from build123d import *

# Parameters (mm, degrees)
SKETCH1_W                                         = 6.35
SKETCH1_H                                         = 9.5
BOSS_EXTRUDE1_DEPTH                               = 5.3
SKETCH2_W                                         = 17.283420288
SKETCH2_H                                         = 7.484
BOSS_EXTRUDE2_DEPTH                               = 3.175
SKETCH3_R                                         = 0.954
CUT_EXTRUDE1_DEPTH                                = 16.91379719
SKETCH4_W                                         = 6.35
SKETCH4_H                                         = 1.008
BOSS_EXTRUDE3_DEPTH                               = 3.175
CHAMFER1_SIZE                                     = 3.175
CHAMFER2_SIZE                                     = 1.5875
CHAMFER3_SIZE                                     = 0.762
CSK_FOR_4_FLAT_HEAD_MACHINE_SCREW_100_D           = 3.4544
CSK_FOR_4_FLAT_HEAD_MACHINE_SCREW_100_CSINK_D     = 5.715
CSK_FOR_4_FLAT_HEAD_MACHINE_SCREW_100_CSINK_ANGLE = 100


with BuildPart() as part:
    # Sketch1 → Boss-Extrude1 (new body)
    with BuildSketch(Plane.XY):
        with Locations((9.429, 0)):
            Rectangle(SKETCH1_W, SKETCH1_H)
    extrude(amount=BOSS_EXTRUDE1_DEPTH)

    # Sketch2 → Boss-Extrude2 (add)
    with BuildSketch(Plane.XY.offset(5.3)):
        with Locations((3.962289856, 0)):
            Rectangle(SKETCH2_W, SKETCH2_H)
    extrude(amount=BOSS_EXTRUDE2_DEPTH)

    # Sketch3 → Cut-Extrude1 (cut, through all)
    with BuildSketch(Plane.XY.offset(8.475)):
        with Locations((-4, 0)):
            Circle(SKETCH3_R)
        with Locations((3.5, 0)):
            Circle(SKETCH3_R)
    extrude(amount=-CUT_EXTRUDE1_DEPTH, mode=Mode.SUBTRACT)

    # Sketch4 → Boss-Extrude3 (add)
    with BuildSketch(Plane.XY.offset(5.3)):
        with Locations((9.429, 4.246)):
            Rectangle(SKETCH4_W, SKETCH4_H)
        with Locations((9.429, -4.246)):
            Rectangle(SKETCH4_W, SKETCH4_H)
    extrude(amount=BOSS_EXTRUDE3_DEPTH)

    # Chamfer1
    # the kernel refuses this chamfer: 3.175 mm, written as the material it adds along each edge
    with BuildSketch(Plane(origin=(6.254, 3.742, 5.3), x_dir=(-0.9996219169112968, -0.027495876610586466, 0), z_dir=(0, 0, 1))) as chamfer1_piece_1_section:
        Polygon((CHAMFER1_SIZE * 0.999621916911, -CHAMFER1_SIZE * 0.0274958766106), (-CHAMFER1_SIZE * 0.0274958766106, -CHAMFER1_SIZE * 0.999621916911), (0, 0), align=None)
    chamfer1_piece_1 = extrude(amount=3.175, mode=Mode.PRIVATE)
    chamfer1_piece_1 = split(chamfer1_piece_1, bisect_by=Plane(origin=(4.881200971, 4.75, 6.8875), z_dir=(0, -1, 0)), keep=Keep.TOP, mode=Mode.PRIVATE)
    add(chamfer1_piece_1)
    with BuildSketch(Plane(origin=(6.254, -3.742, 5.3), x_dir=(-0.9996219169112968, 0.027495876610586324, 0), z_dir=(0, 0, 1))) as chamfer1_piece_2_section:
        Polygon((CHAMFER1_SIZE * 0.999621916911, CHAMFER1_SIZE * 0.0274958766106), (-CHAMFER1_SIZE * 0.0274958766106, CHAMFER1_SIZE * 0.999621916911), (0, 0), align=None)
    chamfer1_piece_2 = extrude(amount=3.175, mode=Mode.PRIVATE)
    chamfer1_piece_2 = split(chamfer1_piece_2, bisect_by=Plane(origin=(4.881200971, -4.75, 6.8875), z_dir=(0, 1, 0)), keep=Keep.TOP, mode=Mode.PRIVATE)
    add(chamfer1_piece_2)

    # Chamfer2
    chamfer2_edges = [part.edges().sort_by_distance(p)[0] for p in [
        (12.604, 4.75, 4.2375),
        (12.604, -4.75, 4.2375),
        (-4.679420288, 3.742, 6.8875),
        (-4.679420288, -3.742, 6.8875),
    ]]
    chamfer(chamfer2_edges, length=CHAMFER2_SIZE)

    # Chamfer3
    chamfer3_edges = [part.edges().sort_by_distance(p)[0] for p in [
        (-0.006460144, -3.742, 5.3),
        (-4.679420288, 1.412102233, 5.3),
        (-3.885670288, 2.94825, 5.3),
        (-3.885670288, -2.94825, 5.3),
        (-4.679420288, -1.412102233, 5.3),
        (-3.046, 0, 5.3),
        (2.546, 0, 5.3),
        (-0.006460144, 3.742, 5.3),
        (6.254, -4.75, 2.65),
        (6.254, 4.75, 2.65),
        (3.583, 4.246, 5.3),
        (3.583, -4.246, 5.3),
        (5.1705, 4.75, 5.3),
        (5.1705, -4.75, 5.3),
    ]]
    chamfer(chamfer3_edges, length=CHAMFER3_SIZE)

    # CSK for #4 Flat Head Machine Screw (100)1 (through all)
    with Locations(Plane.XY.offset(8.475)):
        with Locations((9.429, 0)):
            CounterSinkHole(CSK_FOR_4_FLAT_HEAD_MACHINE_SCREW_100_D / 2, CSK_FOR_4_FLAT_HEAD_MACHINE_SCREW_100_CSINK_D / 2, counter_sink_angle=CSK_FOR_4_FLAT_HEAD_MACHINE_SCREW_100_CSINK_ANGLE)


solid = part.part
Build history of the part. All positions in model axes, mm. A direction names the side the tool comes from. Coordinates: 2 decimals unless noted, no trailing zeros. Order: outer loops, then holes, each group sorted by start corner. A loop starts at its lowest first (then second) coordinate and runs counter-clockwise, first axis right, second up. Notation, with made-up numbers: (-23.75, -22) -> (11.25, -22) arc R26 ccw to (11.25, -8) -> close; hole circle Ø4 at (60.25, 2). An arc over 180 degrees is marked (long way). One line per item, written item: value.
(1) Slice it at B-B, the plane z = 5. List the corners of the cut face in (x, y), plus the area to 3 significant figures.
Checked values:
outline: (6.25, -3.99) -> (7.02, -4.75) -> (11.02, -4.75) -> (12.6, -3.16) -> (12.6, 3.16) -> (11.02, 4.75) -> (7.02, 4.75) -> (6.25, 3.99) -> close; hole circle Ø3.45 at (9.43, 0)
area: 47.9 mm2
(2) Slice it at C-C, the plane z = 7.75. List the corners of the cut face in (x, y).
Checked values:
outline: (-4.68, -2.15) -> (-3.09, -3.74) -> (3.08, -3.74) -> (4.09, -4.75) -> (11.02, -4.75) -> (12.6, -3.16) -> (12.6, 3.16) -> (11.02, 4.75) -> (4.09, 4.75) -> (3.08, 3.74) -> (-3.09, 3.74) -> (-4.68, 2.15) -> (-4.68, 0.67) arc R0.95 cw (long way) to (-4.68, -0.67) -> close; hole circle Ø1.91 at (3.5, 0); hole circle Ø3.99 at (9.43, 0)
(3) Slice it at A-A, the plane y = 0. Count the separate pieces of the cut face and the enclosed holes in it, plus the area to 3 significant figures.
Checked values:
separate pieces: 3
enclosed holes: 0
area: 46.1 mm2
(4) Probe line 1 (X direction, y = 0, z = 2.5); line 2 (X direction, y = 0, z = 6); line 3 (Y direction, x = 1, z = 6.25). List the from-to ranges inside material, lowest first. Write a range as [from, to].
Checked values:
line 1: [6.25, 7.7], [11.16, 12.6]
line 2: [-2.98, 2.48], [4.52, 7.7], [11.16, 12.6]
line 3: [-3.74, 3.74]
(5) Drop flat-ended pins along their axis: pin 1 Ø2.5 at (x, y) = (-4, 0) entering from -Z; pin 2 Ø4 at (y, z) = (0.5, 3) entering from -X; pin 3 Ø0.7 at (x, z) = (-1, 8) entering from +Y. Give the stop position or say it passes through.
Checked values:
pin 1: z = 5.77
pin 2: x = 6.25
pin 3: y = 3.74
(6) Tool access for faces 1 (the flat face through (4, -1, 8.475)), 2 (the flat face through (6.254, 0, 3)), 3 (the flat face through (0, 3.742, 7)): list every direction of +Z, -Z, +X, -X, +Y, -Y with a clear straight run to the whole face (end or side of a thin tool).
Checked values:
face 1: +Z, +X, -X, +Y, -Y
face 2: -Z, -X, +Y, -Y
face 3: +Z, -Z, -X, +Y
(7) Mould opens along Y. For faces 4 (the flat face through (7, 0, 0)), 5 (the cylindrical face through (-3.047, -0.032, 7.285)), 6 (the cylindrical face through (7.78, 0.52, 3.71)), 7 (the flat face through (0, -3.742, 7)) say: pulls with the +Y half, pulls with the -Y half, needs draft (parallel to the pull), parting line crosses it, or undercut.
Checked values:
face 4: needs draft
face 5: undercut
face 6: undercut
face 7: pulls with the -Y half
